```python
from build123d import *

# Parameters (mm, degrees)
F0_W     = 60
F0_H     = 70
F1_DEPTH = 10


with BuildPart() as f1:
    # F0 (on Top) → F1 (new body)
    with BuildSketch(Plane.XY):
        Polygon((-10.705919, 83.133888), (-25.705919, 47.133888), (4.294081, 47.133888), align=None)
        Polygon((-25.705919, 47.133888), (-40.705919, 17.133888), (19.294081, 17.133888), (4.294081, 47.133888), align=None)
        with Locations((-10.705919, -17.866112)):
            Rectangle(F0_W, F0_H)
    extrude(amount=F1_DEPTH)


solid = f1.part
```
CAD build for the part. Positions are in the model's coordinates, mm. Round coordinates to 2 decimals unless told otherwise and drop trailing zeros. Loops run counter-clockwise (first coordinate to the right, second up) from the corner with the lowest first, then second, coordinate; pieces in that order, holes last. Notation, with made-up numbers: (48.5, 64.25) - (58.5, 64.25) arc R20 ccw to (58.5, 89.25) - close; hole circle Ø2 at (36, -26.5). An arc over 180 degrees is marked (long way). Return JSON: item names as keys, results as strings. Group by question number.
Q1. Band-saw the part on C-C on y = 66. Give the cut face in (x, z).
Q2. Drill centre lines: line 1 along Y through (x, z) = (3, 5); line 2 along Y through (x, z) = (-15, 9); line 3 along X through (y, z) = (20, 2). Where is each one in solid material? Low to high. Write a range as [from, to].
Q3. Band-saw the part on A-A on z = 4.5. Give the cut face in (x, y).
Q4. Flat gauge pins, fed straight in: pin 1 Ø3 at (x, z) = (12, 4) entering from +Y; pin 2 Ø1 at (y, z) = (56.5, 4.5) entering from -X; pin 3 Ø2 at (y, z) = (48.5, 3) entering from -X. Where does each tip first touch, or does it go through?
Q5. Band-saw the part on B-B on x = 9.5. Give the cut face in (y, z), plus the area to 3 significant figures.
Solutions:
{
 "1": {"outline": "(-17.85, 0) - (-3.57, 0) - (-3.57, 10) - (-17.85, 10) - close"},
 "2": {"line 1": "y = [-52.87, 50.24]", "line 2": "y = [-52.87, 72.83]", "line 3": "x = [-39.27, 17.86]"},
 "3": {"outline": "(-40.71, -52.87) - (19.29, -52.87) - (19.29, 17.13) - (4.29, 47.13) - (-10.71, 83.13) - (-25.71, 47.13) - (-40.71, 17.13) - close"},
 "4": {"pin 1": "stops at y = 34.72", "pin 2": "stops at x = -22.01", "pin 3": "stops at x = -25.55"},
 "5": {"outline": "(-52.87, 0) - (36.72, 0) - (36.72, 10) - (-52.87, 10) - close", "area": "896 mm^2"}
}
